from build123d import *

# Parameters (mm, degrees)
SKETCH3_W           = 2.5
SKETCH3_H           = 2.5
LPATTERN2_COUNT     = 3
LPATTERN2_PITCH     = 6
SKETCH6_W           = 30
SKETCH6_H           = 13.374164213
CUT_EXTRUDE1_DEPTH  = 35
FILLET1_R           = 5
FILLET2_R           = 5
FILLET3_R           = 5
DOME1_FACE_RADIUS   = 35
DOME1_HEIGHT        = 5
SKETCH8_R           = 9
CUT_EXTRUDE2_DEPTH  = 2.5
SKETCH9_R           = 7.5
BOSS_EXTRUDE1_DEPTH = 32.5
SKETCH10_R          = 5
CUT_EXTRUDE3_DEPTH  = 32.5


with BuildPart() as part:
    # Sketch2 → Revolve1 (revolve)
    with BuildSketch(Plane.XY, mode=Mode.PRIVATE) as revolve1_sk:
        Polygon((0, 0), (0, -10), (23, -10), (23, -70), (35, -70), (35, 0), align=None)
    revolve(revolve1_sk.sketch.rotate(Axis((0, 0, 0), (0, -1, 0)), 90), axis=Axis((0, 0, 0), (0, -1, 0)))

    # Sketch3 → Cut-Revolve2 (revolve, cut)
    with BuildSketch(Plane.XY, mode=Mode.PRIVATE) as cut_revolve2_sk:
        with Locations((33.75, -6.610674558)):
            Rectangle(SKETCH3_W, SKETCH3_H)
    cut_revolve2 = revolve(cut_revolve2_sk.sketch.rotate(Axis((0, 0, 0), (0, -1, 0)), 90), axis=Axis((0, 0, 0), (0, -1, 0)), mode=Mode.SUBTRACT)

    # LPattern2: Cut-Revolve2 ×3
    with Locations(*[(0, -i * LPATTERN2_PITCH, 0) for i in range(1, LPATTERN2_COUNT)]):
        add(cut_revolve2, mode=Mode.SUBTRACT)

    # Sketch6 → Cut-Extrude1 (cut, symmetric)
    with BuildSketch(Plane.XY):
        with Locations((0.25670187, -63.312917893)):
            Rectangle(SKETCH6_W, SKETCH6_H)
    extrude(amount=CUT_EXTRUDE1_DEPTH, both=True, mode=Mode.SUBTRACT)

    # Fillet1
    fillet1_edges = [part.edges().sort_by_distance(p)[0] for p in [
        (-14.74329813, -56.625835787, 24.698230373),
    ]]
    fillet(fillet1_edges, radius=FILLET1_R)

    # Fillet2
    fillet2_edges = [part.edges().sort_by_distance(p)[0] for p in [
        (15.25670187, -56.625835787, 24.355576471),
        (-14.74329813, -56.625835787, -24.698230373),
        (15.25670187, -56.625835787, -24.355576471),
    ]]
    fillet(fillet2_edges, radius=FILLET2_R)

    # Fillet3
    fillet3_edges = [part.edges().sort_by_distance(p)[0] for p in [
        (15.25670187, -70, 24.355576471),
        (-14.74329813, -70, 24.698230373),
        (15.25670187, -70, -24.355576471),
        (-14.74329813, -70, -24.698230373),
    ]]
    fillet(fillet3_edges, radius=FILLET3_R)

    # Dome1: a dome of height H over a round flat face of radius A is a cap of a sphere of radius (A * A + H * H) / (2 * H)
    dome1_r = (DOME1_FACE_RADIUS * DOME1_FACE_RADIUS + DOME1_HEIGHT * DOME1_HEIGHT) / (2 * DOME1_HEIGHT)
    dome1_base = Plane((0, 0, 0), z_dir=(0, 1, 0))
    with Locations(dome1_base.offset(DOME1_HEIGHT - dome1_r)):
        dome1_ball = Sphere(dome1_r, mode=Mode.PRIVATE)
    add(split(dome1_ball, bisect_by=dome1_base, keep=Keep.TOP, mode=Mode.PRIVATE))

    # Sketch8 → Cut-Extrude2 (cut)
    with BuildSketch(Plane(origin=(35, 0, 0), x_dir=(0, 0, -1), z_dir=(1, 0, 0))):
        with Locations((0, -55)):
            Circle(SKETCH8_R)
    cut_extrude2 = extrude(amount=-CUT_EXTRUDE2_DEPTH, mode=Mode.SUBTRACT)

    # Mirror1: Cut-Extrude2 across plane
    add(cut_extrude2.mirror(Plane(origin=(0, 0, 0), x_dir=(0, 0, 1), z_dir=(1, 0, 0))), mode=Mode.SUBTRACT)

    # Sketch9 → Boss-Extrude1 (add, symmetric)
    with BuildSketch(Plane(origin=(0, 0, 0), x_dir=(0, 0, -1), z_dir=(1, 0, 0))):
        with Locations(Location((0, -55, 0), (0, 0, 180))):
            Circle(SKETCH9_R)
    extrude(amount=BOSS_EXTRUDE1_DEPTH, both=True)

    # Sketch10 → Cut-Extrude3 (cut, symmetric)
    with BuildSketch(Plane(origin=(0, 0, 0), x_dir=(0, 0, -1), z_dir=(1, 0, 0))):
        with Locations((0, -55)):
            Circle(SKETCH10_R)
    extrude(amount=CUT_EXTRUDE3_DEPTH, both=True, mode=Mode.SUBTRACT)


solid = part.part
Part model, mm, in its own coordinate system. A direction names the side the tool comes from. Coordinates: 2 decimals unless noted, no trailing zeros. Loops run counter-clockwise (first coordinate to the right, second up) from the corner with the lowest first, then second, coordinate; pieces in that order, holes last. Notation, with made-up numbers: M 48.25,-21.75 L 97.25,-21.75 A24 cw 97.25,-11.75 Z; hole C 17.25,15 d8. An arc over 180 degrees is marked long. Use a Markdown table: item, result. Add a question column.
Q1. Probe L1, parallel to Y at x = -33.1, z = 0; L2, parallel to Y at x = 34.3, z = 0; L3, parallel to Y at x = 4.5, z = 0. List the from-to ranges inside material, lowest first.
Q2. Mould opens along X. For faces 5 (the flat face through (-32.5, -51, 4)), 6 (the flat face through (23.2, -7.861, -23.2)), 7 (the flat face through (0, -56.626, 28)) say: +X half, -X half, draft (parallel to the pull), parting line (faces both ways), or undercut.
Q3. Which spindle directions (+Z, -Z, +X, -X, +Y, -Y) get a long thin tool onto all of the face, cutting with end or side? Do faces 1 (the cylindrical face through (13.8, -58.1, 25.2)), 2 (the flat face through (15.257, -63, -24)), 3 (the cylindrical face through (-9.76, -6.59, 31)), 4 (the cylindrical face through (16.683, -68.496, -23.342)). Say none if no direction does.
Q4. Cut at A-A (x = 0). Give the number of separate pieces and of enclosed holes in the cut face, and give its area (3 significant figures).
Q5. Cut at B-B (y = -55). Write the cut outline in (x, z).
Q6. Pin check, flat tips, straight feed: P1, Ø5, axis at x = 0, z = -5.5, coming from the -Y side; P2, Ø16, axis at x = 4, z = 28.5, coming from the -Y side; P3, Ø1.5, axis at x = 18, z = -22.5, coming from the +Y side; P4, Ø6, axis at y = -55, z = 0, coming from the +X side. Stop position of each tip, or through.
Worked out:
| question | item | result |
|---|---|---|
| 1 | L1 | y = -70 to -64, -46 to -19.86, -17.36 to -13.86, -11.36 to -7.86, -5.36 to 0.54 |
| 1 | L2 | y = -70 to -64, -46 to -19.86, -17.36 to -13.86, -11.36 to -7.86, -5.36 to 0.2 |
| 1 | L3 | y = -62.5 to -60, -50 to -47.5, -10 to 4.92 |
| 2 | face 5 | -X half |
| 2 | face 6 | draft |
| 2 | face 7 | undercut |
| 3 | face 1 | +Z, -Y |
| 3 | face 2 | -Z, -Y |
| 3 | face 3 | none |
| 3 | face 4 | +Z, -Z, -Y |
| 4 | separate pieces | 2 |
| 4 | enclosed holes | 1 |
| 4 | area | 2,110 mm2 |
| 5 | outline | M -33.82,-9 A35 ccw 33.82,-9 L 32.5,-9 L 32.5,-5 L -32.5,-5 L -32.5,-9 Z; M -33.82,9 L -32.5,9 L -32.5,5 L 32.5,5 L 32.5,9 L 33.82,9 A35 ccw Z; hole M -21.74,-7.5 A23 ccw 21.74,-7.5 Z; hole M -21.74,7.5 L 21.74,7.5 A23 ccw Z |
| 6 | P1 | stops at y = -61.87 |
| 6 | P2 | stops at y = -56.94 |
| 6 | P3 | stops at y = 1.81 |
| 6 | P4 | passes through |
